Design review of the part built by this model. Coordinates are the model's own, in mm. A direction names the side the tool comes from. Coordinates: 2 decimals unless noted, no trailing zeros. Loops run counter-clockwise (first coordinate to the right, second up) from the corner with the lowest first, then second, coordinate; pieces in that order, holes last. Notation, with made-up numbers: (66, 2.5) - (71, 2.5) arc R31 cw to (71, 36.5) - close; hole circle Ø9 at (18.25, 73). An arc over 180 degrees is marked (long way). Return JSON: item names as keys, results as strings. Group by question number.
from build123d import *

# Parameters (mm, degrees)
SKETCH2_W                  = 82.738044028
SKETCH2_H                  = 243.598411898
BOSS_EXTRUDE1_DEPTH        = 3.175
BOSS_EXTRUDE2_DEPTH        = 243.598412
SKETCH3_W                  = 13.462
SKETCH3_H                  = 111.125
CUT_EXTRUDE1_DEPTH         = 16.816415828
CUT_EXTRUDE1_DEPTH_BACK    = 12.72988093
FILLET1_R                  = 6.35
SKETCH4_W                  = 57.955870979
SKETCH4_H                  = 238.518411898
CUT_EXTRUDE2_DEPTH         = 4.175
FILLET2_R                  = 6.35
F_6_0_204_DIAMETER_HOLE1_D = 5.1816
CUT_EXTRUDE3_DEPTH         = 11.207293294


with BuildPart() as part:
    # Sketch2 → Boss-Extrude1 (new body)
    with BuildSketch(Plane.XY):
        with Locations((870.137648104, 6053.851709568)):
            Rectangle(SKETCH2_W, SKETCH2_H)
    extrude(amount=BOSS_EXTRUDE1_DEPTH)

    # Sketch5 → Boss-Extrude2 (add, through all)
    with BuildSketch(Plane(origin=(0, 6175.650915517, 0), x_dir=(1, 0, 0), z_dir=(0, 1, 0))):
        Polygon((828.76862609, -3.175), (843.956978058, -13.382293294), (848.647124982, -12.555293847), (846.99312609, -3.175), align=None)
    extrude(amount=-BOSS_EXTRUDE2_DEPTH)

    # Sketch3 → Cut-Extrude1 (cut, two sides)
    with BuildSketch(Plane(origin=(1789.989771594, 0, -153.428812844), x_dir=(-0.984807753, 0, 0.173648178), z_dir=(-0.173648178, 0, -0.984807753))) as cut_extrude1_sk:
        with Locations((967.081003168, 6016.190003619)):
            Rectangle(SKETCH3_W, SKETCH3_H)
    extrude(amount=CUT_EXTRUDE1_DEPTH, mode=Mode.SUBTRACT)
    extrude(cut_extrude1_sk.sketch, amount=-CUT_EXTRUDE1_DEPTH_BACK, mode=Mode.SUBTRACT)

    # Fillet1
    fillet1_edges = [part.edges().sort_by_distance(p)[0] for p in [
        (843.054051922, 6071.752503619, 6.667107565),
        (843.054051922, 5960.627503619, 6.667107565),
    ]]
    fillet(fillet1_edges, radius=FILLET1_R)

    # Sketch4 → Cut-Extrude2 (cut, through all)
    with BuildSketch(Plane.XY.offset(3.175)):
        with Locations((876.178734629, 6051.311709568)):
            Rectangle(SKETCH4_W, SKETCH4_H)
    extrude(amount=-CUT_EXTRUDE2_DEPTH, mode=Mode.SUBTRACT)

    # Fillet2
    fillet2_edges = [part.edges().sort_by_distance(p)[0] for p in [
        (905.156670118, 6170.570915517, 1.5875),
        (847.200799139, 6170.570915517, 1.5875),
    ]]
    fillet(fillet2_edges, radius=FILLET2_R)

    # #6 (0.204) Diameter Hole1 (through all)
    with Locations(Plane(origin=(0, 0, 0), x_dir=(-1, 0, 0), z_dir=(0, 0, -1))):
        with Locations((-833.65812609, 6161.363415517), (-833.65812609, 6142.313415517), (-833.65812609, 5946.340003619)):
            Hole(F_6_0_204_DIAMETER_HOLE1_D / 2)

    # Sketch8 → Cut-Extrude3 (cut, through all)
    with BuildSketch(Plane.XY.offset(3.175)):
        with BuildLine():
            Line((833.65812609, 6156.283415517), (828.76862609, 6156.283415517))
            ThreePointArc((828.76862609, 6156.283415517), (823.68862609, 6161.363415517), (828.76862609, 6166.443415517))
            Line((828.76862609, 6166.443415517), (833.65812609, 6166.443415517))
            ThreePointArc((833.65812609, 6166.443415517), (838.73812609, 6161.363415517), (833.65812609, 6156.283415517))
        make_face()
        with BuildLine():
            Line((833.65812609, 6137.233415517), (828.76862609, 6137.233415517))
            ThreePointArc((828.76862609, 6137.233415517), (823.68862609, 6142.313415517), (828.76862609, 6147.393415517))
            Line((828.76862609, 6147.393415517), (833.65812609, 6147.393415517))
            ThreePointArc((833.65812609, 6147.393415517), (838.73812609, 6142.313415517), (833.65812609, 6137.233415517))
        make_face()
        with BuildLine():
            Line((833.65812609, 5941.260003619), (828.76862609, 5941.260003619))
            ThreePointArc((828.76862609, 5941.260003619), (823.68862609, 5946.340003619), (828.76862609, 5951.420003619))
            Line((828.76862609, 5951.420003619), (833.65812609, 5951.420003619))
            ThreePointArc((833.65812609, 5951.420003619), (838.73812609, 5946.340003619), (833.65812609, 5941.260003619))
        make_face()
    extrude(amount=CUT_EXTRUDE3_DEPTH, mode=Mode.SUBTRACT)


solid = part.part
Item 1: Add section C-C (x = 901.5). State the section outline as (y, z) points (3 decimals), then the cut area to 3 significant figures.
Item 2: Add section B-B (x = 881). State the section outline as (y, z) points (3 decimals), then the cut area to 3 significant figures.
Item 3: Draft analysis for pull direction X (two halves, no side actions). For faces 1 (the face through (836.26, 6122.21, 8.21)), 2 (the face through (833.096, 6139.784, 1.61)), 3 (the face through (903.35, 6168.66, 1.57)), 4 (the face through (846.269, 6055.557, 12.975)), state which applies: pulls with the +X half, pulls with the -X half, needs draft (parallel to the pull), parting line crosses it, or undercut.
Item 4: For faces 5 (the face through (839.632, 5948.819, 10.475)), 6 (the face through (849.11, 6168.76, 1.57)), 7 (the face through (838.737, 5946.452, 5.734)), list the 3-axis set-ups (+Z, -Z, +X, -X, +Y, -Y) from which the entire face can be reached by the end or side of a thin tool; tool diameter is ignored.
Item 5: For P1, Ø6, axis at x = 854.5, y = 6036, coming from the +Z side; P2, Ø1, axis at x = 866.5, z = 2, coming from the -Y side; P3, Ø3, axis at y = 6026, z = 7.5, coming from the -X side; P4, Ø4, axis at y = 6128.5, z = 6, coming from the +X side, all flat-tipped, find the tip position at first contact; note any pin that passes through.
Item 6: To check wall thickness, follow line 1 (X direction, y = 6143, z = 1); line 2 (Y direction, x = 899, z = 0.75); line 3 (Y direction, x = 839, z = 9). State the ranges of each line that lie inside material, in increasing order. Write a range as from..to.
Item 7: Add section A-A (y = 6087). State the section outline as (x, z) points (3 decimals), then the cut area to 3 significant figures.
Answers below:
{
 "1": {"outline": "(6169.971, 0) - (6175.651, 0) - (6175.651, 3.175) - (6169.971, 3.175) - close", "area": "18.0 mm^2"},
 "2": {"outline": "(6170.571, 0) - (6175.651, 0) - (6175.651, 3.175) - (6170.571, 3.175) - close", "area": "16.1 mm^2"},
 "3": {"face 1": "pulls with the -X half", "face 2": "undercut", "face 3": "undercut", "face 4": "pulls with the +X half"},
 "4": {"face 5": "+Z, -X, +Y, -Y", "face 6": "-Z, -Y", "face 7": "+Z, -X"},
 "5": {"P1": "passes through", "P2": "stops at y = 6170.57", "P3": "stops at x = 842.94", "P4": "stops at x = 847.84"},
 "6": {"line 1": "x = 828.77..831.16, 836.16..847.2, 905.16..911.51", "line 2": "y = 6170.57..6175.65", "line 3": "y = 5932.05..5960.94, 6071.44..6175.65"},
 "7": {"outline": "(828.769, 0) - (847.201, 0) - (847.201, 3.175) - (846.993, 3.175) - (848.647, 12.555) - (843.957, 13.382) - (828.769, 3.175) - close; (905.157, 0) - (911.507, 0) - (911.507, 3.175) - (905.157, 3.175) - close", "area": "194 mm^2"}
}
